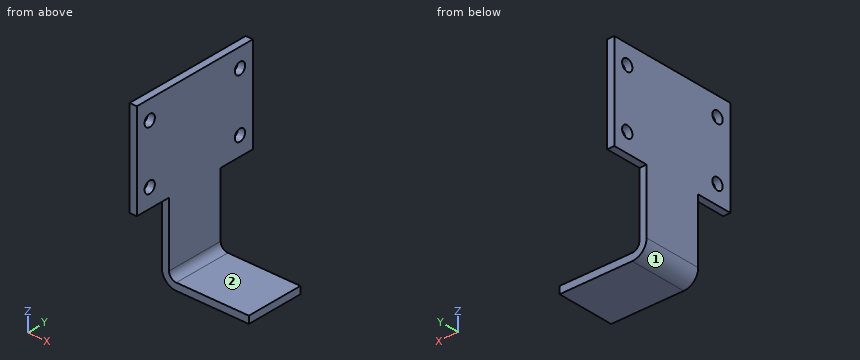
Autodesk Inventor part; units mm, degrees
ref_plane "YZ Plane" through (0, 0, 0) normal (1, 0, 0) x (0, 1, 0)
ref_plane "XZ Plane" through (0, 0, 0) normal (0, 1, 0) x (-1, 0, 0)
ref_plane "XY Plane" through (0, 0, 0) normal (0, 0, 1) x (1, 0, 0)
sketch "Sketch1" plane through (0, 0, 0) normal (0, 1, 0) x (-1, 0, 0)
  line L0 (-38.1, 0) -> (0, 0)
  line L1 (0, 0) -> (0, 76.2)
  line L2 (0, 76.2) -> (-3.175, 76.2)
  line L3 (-38.1, 0) -> (-38.1, 3.175)
  line L4 (-38.1, 3.175) -> (-3.175, 3.175)
  line L5 (-3.175, 3.175) -> (-3.175, 76.2)
  dimension "d0" = 38.1
  dimension "d1" = 76.2
  dimension "d2" = 3.175
extrude "Extrusion1" add sketch "Sketch1" along normal blind 57.15
sketch "Sketch2" plane through (38.1, 0, 3.175) normal (1, 0, 0) x (0, 0, -1)
  line L0 (3.175, 57.15) -> (-31.115, 57.15)
  line L1 (-31.115, 57.15) -> (-31.115, 41.275)
  line L2 (-31.115, 41.275) -> (3.175, 41.275)
  line L3 (3.175, 41.275) -> (3.175, 57.15)
  line L4 (3.175, 0) -> (-31.115, 0)
  line L5 (-31.115, 0) -> (-31.115, 15.875)
  line L6 (-31.115, 15.875) -> (3.175, 15.875)
  line L7 (3.175, 15.875) -> (3.175, 0)
  line L8 (-64.77, 50.8) -> (-39.37, 50.8) construction
  line L9 (-39.37, 50.8) -> (-39.37, 6.35) construction
  line L10 (-39.37, 6.35) -> (-64.77, 6.35) construction
  line L11 (-64.77, 6.35) -> (-64.77, 50.8) construction
  line L12 (-52.07, 50.8) -> (-52.07, 57.15) construction
  line L13 (-52.07, 6.35) -> (-52.07, 0) construction
  line L14 (-73.025, 57.15) -> (0, 57.15) construction
  line L15 (0, 0) -> (-73.025, 0) construction
  circle A0 centre (-39.37, 50.8) radius 2.54
  circle A1 centre (-64.77, 50.8) radius 2.54
  circle A2 centre (-39.37, 6.35) radius 2.54
  circle A3 centre (-64.77, 6.35) radius 2.54
  line L16 (-73.025, 0) -> (-73.025, 57.15) construction
  line L17 (-39.37, 50.8) -> (-31.115, 50.8) construction
  line L18 (-64.77, 50.8) -> (-73.025, 50.8) construction
  dimension "d5" = 25.4
  dimension "d6" = 44.45
  dimension "d8" = 5.08
  dimension "d9" = 25.4
  dimension "d10" = 41.91
extrude "Extrusion2" cut sketch "Sketch2" against normal through all
fillet "Fillet1" radius 3.175 1 edges at (3.175, 28.575, 3.175)
fillet "Fillet1" radius 6.35 1 edges at (0, 28.575, 0)
properties part number "motor mount" material "Aluminum 6061"
Read the model definition and answer for the solid it produces. Units are mm, in the model's axes. Face numbers are marked on the shaded views. A direction names the side the tool comes from. Round coordinates to 2 decimals unless told otherwise and drop trailing zeros. Write each loop counter-clockwise with the first axis right and the second up, starting at its lowest first coordinate (ties: lowest second). Pieces come first, ordered by that corner, then holes. Notation, with made-up numbers: M 60,41 L 88,41 A23 ccw 88,64 Z; hole C -28,12.25 d8. An arc over 180 degrees is marked long. One line per item, written item: value.
Q1. Find section A-A on y = 50.8. Write down the section's boundary in (x, z) (3 decimals).
Data:
outline: M 0,34.29 L 3.175,34.29 L 3.175,40.005 L 0,40.005 Z; M 0,45.085 L 3.175,45.085 L 3.175,65.405 L 0,65.405 Z; M 0,70.485 L 3.175,70.485 L 3.175,76.2 L 0,76.2 Z
Q2. Straight lines are drawn through the part: line 1 (X direction, y = 13, z = 70) (3 decimals); line 2 (Y direction, x = 18.5, z = 3) (3 decimals); line 3 (Z direction, x = 6, y = 22). For each, find the intervals that lie inside material, in ascending order. Write a range as [from, to].
Data:
line 1: [0, 3.175]
line 2: [15.875, 41.275]
line 3: [0.01, 3.19]
Q3. Find section D-D on x = 18. Write down the section's boundary in (y, z) (3 decimals), plus the area to 3 significant figures.
Data:
outline: M 15.875,0 L 41.275,0 L 41.275,3.175 L 15.875,3.175 Z
area: 80.6 mm2
Q4. Which of the six approach directions +Z, -Z, +X, -X, +Y, -Y give full straight-line access (tool end or side, diameter ignored) to the marked faces 1 and 2?
Data:
face 1: -Z, -X, +Y, -Y
face 2: +Z, +X, +Y, -Y
Q5. Find section C-C on y = 25.5. Write down the section's boundary in (x, z) (3 decimals), plus the area to 3 significant figures.
Data:
outline: M 0,6.35 A6.35 ccw 6.35,0 L 38.1,0 L 38.1,3.175 L 6.35,3.175 A3.175 cw 3.175,6.35 L 3.175,76.2 L 0,76.2 Z
area: 346 mm2
Q6. Find section B-B on z = 43.5. Write down the section's boundary in (x, y) (3 decimals), plus the area to 3 significant figures.
Data:
outline: M 0,0 L 3.175,0 L 3.175,3.996 L 0,3.996 Z; M 0,8.704 L 3.175,8.704 L 3.175,48.446 L 0,48.446 Z; M 0,53.154 L 3.175,53.154 L 3.175,57.15 L 0,57.15 Z
area: 152 mm2
Q7. Flat-ended cylindrical pins translate along their axes: pin 1 Ø8 at (y, z) = (6.35, 67.945) entering from +X (3 decimals); pin 2 Ø7.5 at (x, y) = (27.5, 26) entering from +Z (3 decimals); pin 3 Ø1.6 at (x, y) = (1, 8.5) entering from -Z. Find the tip coordinate at first contact, or state that the pin passes through.
Data:
pin 1: x = 3.175
pin 2: z = 3.175
pin 3: z = 34.29
